from build123d import *

# Parameters (mm, degrees)
F0_W     = 38.1
F0_H     = 19.05
F1_DEPTH = 25.4
F2_SIZE  = 6.35
F3_W     = 63.5
F3_H     = 19.05
F4_DEPTH = 88.9


with BuildPart() as f1:
    # F0 (on Top) → F1 (new body)
    with BuildSketch(Plane.XY):
        with BuildLine():
            Line((30.0978315473, 52.679737395), (7.8728315473, 52.679737395))
            Line((7.8728315473, 52.679737395), (7.8728315473, 20.929737395))
            Line((7.8728315473, 20.929737395), (45.9728315473, 20.929737395))
            Line((45.9728315473, 20.929737395), (45.9728315473, 36.804737395))
            Line((45.9728315473, 36.804737395), (36.4478315473, 36.804737395))
            ThreePointArc((36.4478315473, 36.804737395), (25.6077034867, 32.3146093345), (30.0978315473, 43.154737395))
            Line((30.0978315473, 43.154737395), (30.0978315473, 52.679737395))
        make_face()
        with BuildLine():
            Line((45.9728315473, 52.679737395), (30.0978315473, 52.679737395))
            Line((30.0978315473, 52.679737395), (30.0978315473, 43.154737395))
            ThreePointArc((30.0978315473, 43.154737395), (34.5879596078, 41.2948654556), (36.4478315473, 36.804737395))
            Line((36.4478315473, 36.804737395), (45.9728315473, 36.804737395))
            Line((45.9728315473, 36.804737395), (45.9728315473, 52.679737395))
        make_face()
        with BuildLine():
            Line((7.8728315473, 52.679737395), (-14.3521684527, 52.679737395))
            Line((-14.3521684527, 52.679737395), (-14.3521684527, 43.154737395))
            ThreePointArc((-14.3521684527, 43.154737395), (-9.8620403922, 41.2948654556), (-8.0021684527, 36.804737395))
            ThreePointArc((-8.0021684527, 36.804737395), (-14.3521684527, 30.454737395), (-20.7021684527, 36.804737395))
            Line((-20.7021684527, 36.804737395), (-30.2271684527, 36.804737395))
            Line((-30.2271684527, 36.804737395), (-30.2271684527, 20.929737395))
            Line((-30.2271684527, 20.929737395), (7.8728315473, 20.929737395))
            Line((7.8728315473, 20.929737395), (7.8728315473, 52.679737395))
        make_face()
        with BuildLine():
            Line((-14.3521684527, 52.679737395), (-30.2271684527, 52.679737395))
            Line((-30.2271684527, 52.679737395), (-30.2271684527, 36.804737395))
            Line((-30.2271684527, 36.804737395), (-20.7021684527, 36.804737395))
            ThreePointArc((-20.7021684527, 36.804737395), (-18.8422965133, 41.2948654556), (-14.3521684527, 43.154737395))
            Line((-14.3521684527, 43.154737395), (-14.3521684527, 52.679737395))
        make_face()
        with BuildLine():
            Line((45.9728315473, -48.920262605), (45.9728315473, -33.045262605))
            Line((45.9728315473, -33.045262605), (36.4478315473, -33.045262605))
            ThreePointArc((36.4478315473, -33.045262605), (34.5879596078, -37.5353906655), (30.0978315473, -39.395262605))
            Line((30.0978315473, -39.395262605), (30.0978315473, -48.920262605))
            Line((30.0978315473, -48.920262605), (45.9728315473, -48.920262605))
        make_face()
        with BuildLine():
            Line((45.9728315473, 1.879737395), (7.8728315473, 1.879737395))
            Line((7.8728315473, 1.879737395), (7.8728315473, -48.920262605))
            Line((7.8728315473, -48.920262605), (30.0978315473, -48.920262605))
            Line((30.0978315473, -48.920262605), (30.0978315473, -39.395262605))
            ThreePointArc((30.0978315473, -39.395262605), (25.6077034867, -28.5551345444), (36.4478315473, -33.045262605))
            Line((36.4478315473, -33.045262605), (45.9728315473, -33.045262605))
            Line((45.9728315473, -33.045262605), (45.9728315473, 1.879737395))
        make_face()
        with BuildLine():
            Line((-20.7021684527, -33.045262605), (-30.2271684527, -33.045262605))
            Line((-30.2271684527, -33.045262605), (-30.2271684527, -48.920262605))
            Line((-30.2271684527, -48.920262605), (-14.3521684527, -48.920262605))
            Line((-14.3521684527, -48.920262605), (-14.3521684527, -39.395262605))
            ThreePointArc((-14.3521684527, -39.395262605), (-18.8422965133, -37.5353906655), (-20.7021684527, -33.045262605))
        make_face()
        with BuildLine():
            Line((7.8728315473, 1.879737395), (-30.2271684527, 1.879737395))
            Line((-30.2271684527, 1.879737395), (-30.2271684527, -33.045262605))
            Line((-30.2271684527, -33.045262605), (-20.7021684527, -33.045262605))
            ThreePointArc((-20.7021684527, -33.045262605), (-14.3521684527, -26.695262605), (-8.0021684527, -33.045262605))
            ThreePointArc((-8.0021684527, -33.045262605), (-9.8620403922, -37.5353906655), (-14.3521684527, -39.395262605))
            Line((-14.3521684527, -39.395262605), (-14.3521684527, -48.920262605))
            Line((-14.3521684527, -48.920262605), (7.8728315473, -48.920262605))
            Line((7.8728315473, -48.920262605), (7.8728315473, 1.879737395))
        make_face()
        with Locations((-11.1771684527, 11.404737395)):
            Rectangle(F0_W, F0_H)
        with Locations((26.9228315473, 11.404737395)):
            Rectangle(F0_W, F0_H)
    extrude(amount=F1_DEPTH)

    # F2
    f2_edges = [f1.edges().sort_by_distance(p)[0] for p in [
        (7.872832, 52.679737, 25.4),
        (-30.227168, 1.879737, 25.4),
        (7.872832, -48.920263, 25.4),
        (45.972832, 1.879737, 25.4),
    ]]
    chamfer(f2_edges, length=F2_SIZE)

    # F3 (on face) → F4 (join)
    with BuildSketch(Plane.XY.offset(25.4)):
        with Locations((7.8728315473, -7.645262605)):
            Rectangle(F3_W, F3_H)
    extrude(amount=F4_DEPTH)


solid = f1.part
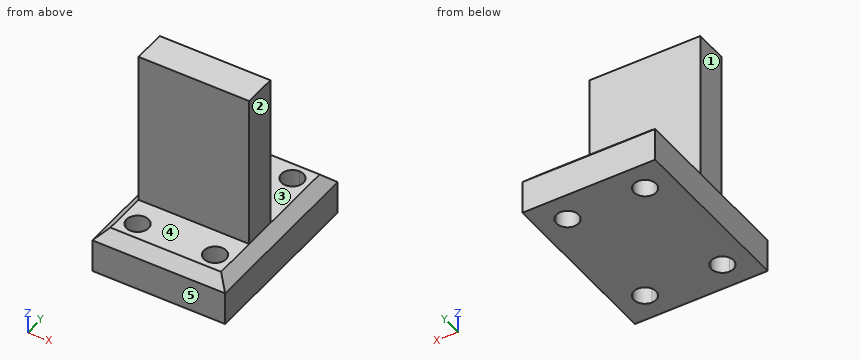
Design review of the part built by this model. Coordinates are the model's own, in mm. Face numbers are marked on the shaded views. A direction names the side the tool comes from. Round coordinates to 2 decimals unless told otherwise and drop trailing zeros. Write each loop counter-clockwise with the first axis right and the second up, starting at its lowest first coordinate (ties: lowest second). Pieces come first, ordered by that corner, then holes.
Item 1: Consider section D-D on y = -35. Give the boundary of the cut face in (x, z), and give its area (3 significant figures).
Item 2: Consider section B-B on z = 21.5. Give the boundary of the cut face in (x, y), and give its area (3 significant figures).
Item 3: For pin 1 Ø22 at (x, y) = (7, 21) entering from +Z; pin 2 Ø14.5 at (x, y) = (30.1, 36.8) entering from -Z; pin 3 Ø9.5 at (y, z) = (-8, 90.5) entering from -X; pin 4 Ø1.5 at (x, z) = (-4.5, 71) entering from -Y, all flat-tipped, find the tip position at first contact; note any pin that passes through.
Item 4: Consider section A-A on y = -4. Give the boundary of the cut face in (x, z).
Item 5: Wall thickness on L1, parallel to Y at x = 35, z = 84; L2, parallel to Z at x = 38, y = -38; L3, parallel to X at y = -1, z = 29: over which ranges is each line inside the solid? List them lowest first.
Item 6: For the marked faces 1, 2, 3, 4 and 5, list the 3-axis set-ups (+Z, -Z, +X, -X, +Y, -Y) from which the entire face can be reached by the end or side of a thin tool; tool diameter is ignored.
Item 7: Consider section C-C on x = -3. Give the boundary of the cut face in (y, z), and give its area (3 significant figures).
Check values:
1. outline: (-30.23, 0) - (-20.39, 0) - (-20.39, 25.4) - (-23.88, 25.4) - (-30.23, 19.05) - close; (-8.31, 0) - (24.06, 0) - (24.06, 25.4) - (-8.31, 25.4) - close; (36.14, 0) - (45.97, 0) - (45.97, 19.05) - (39.62, 25.4) - (36.14, 25.4) - close
1. area: 1,280 mm2
2. outline: (-27.78, -46.47) - (43.52, -46.47) - (43.52, 50.23) - (-27.78, 50.23) - close; hole circle Ø12.7 at (-14.35, -33.05); hole circle Ø12.7 at (-14.35, 36.8); hole circle Ø12.7 at (30.1, -33.05); hole circle Ø12.7 at (30.1, 36.8)
2. area: 6,390 mm2
3. pin 1: stops at z = 25.4
3. pin 2: stops at z = 0
3. pin 3: stops at x = -23.88
3. pin 4: stops at y = -17.17
4. outline: (-30.23, 0) - (45.97, 0) - (45.97, 19.05) - (39.62, 25.4) - (39.62, 114.3) - (-23.88, 114.3) - (-23.88, 25.4) - (-30.23, 19.05) - close
5. L1: y = -17.17 to 1.88
5. L2: z = 0 to 25.4
5. L3: x = -23.88 to 39.62
6. face 1: +Z, -X, +Y, -Y
6. face 2: +Z, +X, +Y, -Y
6. face 3: +Z, +X, -X, +Y
6. face 4: +Z, +X, -X, -Y
6. face 5: +Z, -Z, +X, -X, -Y
7. outline: (-48.92, 0) - (52.68, 0) - (52.68, 19.05) - (46.33, 25.4) - (1.88, 25.4) - (1.88, 114.3) - (-17.17, 114.3) - (-17.17, 25.4) - (-42.57, 25.4) - (-48.92, 19.05) - close
7. area: 4,230 mm2
